Build history of the part. All positions in model axes, mm. A direction names the side the tool comes from. Give positions to 0.01 mm unless a question says otherwise; leave off trailing zeros. Write each loop counter-clockwise with the first axis right and the second up, starting at its lowest first coordinate (ties: lowest second). Pieces come first, ordered by that corner, then holes.
from build123d import *

# Parameters (mm, degrees)
SKETCH1_R               = 9.55
TUBEINTERFACE1_DEPTH    = 5
SKETCH3_R               = 10.922
BODY_DEPTH              = 20.3
BODYCHAMFER_SIZE        = 0.2
SKETCH4_W               = 10
SKETCH4_H               = 75
FLATS_DEPTH             = 12.7
SKETCH5_R               = 7.9375
MOUNTTHREAD1_DEPTH      = 12.7
MOUNTTHREADCHAMFER_SIZE = 1.2
SKETCH17_W              = 2.8
SKETCH17_H              = 5
SKETCH8_R               = 3.5
THRUBORE_DEPTH          = 42.019265815
THRUBORE2_DEPTH         = 38
SKETCH16_R              = 4.639
PORT2_DEPTH             = 10.922
PORT2_DRAFT             = -2
SKETCH26_W              = 2.2
SKETCH26_H              = 0.0127


with BuildPart() as part:
    # Sketch1 → TubeInterface1 (new body)
    with BuildSketch(Plane.XY):
        Circle(SKETCH1_R)
    extrude(amount=TUBEINTERFACE1_DEPTH)

    # Sketch3 → Body (add)
    with BuildSketch(Plane.XY.offset(5)):
        Circle(SKETCH3_R)
    extrude(amount=BODY_DEPTH)

    # BodyChamfer
    bodychamfer_edges = [part.edges().sort_by_distance(p)[0] for p in [
        (-10.922, 0, 25.3),
    ]]
    chamfer(bodychamfer_edges, length=BODYCHAMFER_SIZE)

    # Sketch4 → Flats (cut)
    with BuildSketch(Plane.XY.offset(25.3)):
        with Locations((-14.5, 0)):
            Rectangle(SKETCH4_W, SKETCH4_H)
        with Locations((14.5, 0)):
            Rectangle(SKETCH4_W, SKETCH4_H)
    extrude(amount=-FLATS_DEPTH, mode=Mode.SUBTRACT)

    # Sketch5 → MountThread1 (add)
    with BuildSketch(Plane.XY.offset(25.3)):
        Circle(SKETCH5_R)
    extrude(amount=MOUNTTHREAD1_DEPTH)

    # MountThreadChamfer
    mountthreadchamfer_edges = [part.edges().sort_by_distance(p)[0] for p in [
        (-7.9375, 0, 38),
    ]]
    chamfer(mountthreadchamfer_edges, length=MOUNTTHREADCHAMFER_SIZE)

    # Sketch17 → Cut-Revolve1 (revolve, cut)
    with BuildSketch(Plane(origin=(0, 0, 0), x_dir=(0, 0, -1), z_dir=(1, 0, 0)), mode=Mode.PRIVATE) as cut_revolve1_sk:
        with Locations((-28.9, 9.5)):
            Rectangle(SKETCH17_W, SKETCH17_H)
    revolve(cut_revolve1_sk.sketch.rotate(Axis((0, 0, 0), (0, 0, 1)), 119.564121408), axis=Axis((0, 0, 0), (0, 0, 1)), mode=Mode.SUBTRACT)

    # Sketch8 → ThruBore (cut, through all)
    with BuildSketch(Plane.XY):
        Circle(SKETCH8_R)
    extrude(amount=THRUBORE_DEPTH, mode=Mode.SUBTRACT)

    # Sketch21 → ThruBore2 (cut)
    with BuildSketch(Plane.XY.offset(38)):
        Polygon((3.2, -1.847520861), (3.2, 1.847520861), (0, 3.695041723), (-3.2, 1.847520861), (-3.2, -1.847520861), (0, -3.695041723), align=None)
    extrude(amount=-THRUBORE2_DEPTH, mode=Mode.SUBTRACT)

    # Sketch25 → Chamfer1 (revolve, cut)
    with BuildSketch(Plane(origin=(0, 0, 0), x_dir=(0, 0, -1), z_dir=(1, 0, 0)), mode=Mode.PRIVATE) as chamfer1_sk:
        Polygon((-38, 3.7), (-36, 1.7), (-38, 1.7), align=None)
        Polygon((-38, -3.7), (-36, -1.7), (-38, -1.7), align=None)
    revolve(chamfer1_sk.sketch.rotate(Axis((0, 0, 23.920180356), (0, 0, -1)), 240.435878592), axis=Axis((0, 0, 23.920180356), (0, 0, -1)), mode=Mode.SUBTRACT)


with BuildPart() as port2_tool:
    # Sketch16 → Port2 (with draft: the straight prism first)
    with BuildSketch(Plane(origin=(0, 10.922, 15.05), x_dir=(1, 0, 0), z_dir=(0, 1, 0))):
        with Locations((0, 1.25)):
            Circle(SKETCH16_R)
    extrude(amount=-PORT2_DEPTH)
    # Port2: the draft: its side faces are tilted about the plane it starts from
    port2_sides = [port2_tool.faces().sort_by_distance(p)[0] for p in [
        (-4.639, 5.461, 13.8),
    ]]
    draft(port2_sides, Plane(origin=(0, 10.922, 15.05), x_dir=(1, 0, 0), z_dir=(0, 1, 0)), PORT2_DRAFT)


with BuildPart() as part_1:
    add(part.part)

    # Port2: cut by port2_tool
    add(port2_tool.part, mode=Mode.SUBTRACT)

    # Sketch22 → PortChamfer (revolve, cut)
    with BuildSketch(Plane(origin=(0, 0, 0), x_dir=(0, 0, -1), z_dir=(1, 0, 0)), mode=Mode.PRIVATE) as portchamfer_sk:
        Polygon((-15.8, 10.922), (-19.5, 10.922), (-15.8, 7.222), align=None)
    revolve(portchamfer_sk.sketch.rotate(Axis((0, 0, 13.8), (0, -1, 0)), 90), axis=Axis((0, 0, 13.8), (0, -1, 0)), mode=Mode.SUBTRACT)

    # Sketch23 → RodCoverCrimp (revolve, cut)
    with BuildSketch(Plane(origin=(0, 0, 0), x_dir=(0, 0, -1), z_dir=(1, 0, 0)), mode=Mode.PRIVATE) as rodcovercrimp_sk:
        Polygon((-7.5, 13.6), (-5, 13.6), (-5, 10.2), (-5.5, 10.2), (-7.1, 8.6), (-7.5, 8.6), align=None)
    revolve(rodcovercrimp_sk.sketch.rotate(Axis((0, 0, 0), (0, 0, -1)), 90), axis=Axis((0, 0, 0), (0, 0, -1)), mode=Mode.SUBTRACT)

    # Sketch24 → TubeInterfaceCrimp (revolve, cut)
    with BuildSketch(Plane(origin=(0, 0, 0), x_dir=(0, 0, -1), z_dir=(1, 0, 0)), mode=Mode.PRIVATE) as tubeinterfacecrimp_sk:
        with BuildLine():
            Line((-5, 14.7), (-5, 8.9))
            ThreePointArc((-5, 8.9), (-4.912132034, 8.687867966), (-4.7, 8.6))
            Line((-4.7, 8.6), (-4.1, 8.6))
            Line((-4.1, 8.6), (-3.15, 9.55))
            Line((-3.15, 9.55), (-1, 9.55))
            Line((-1, 9.55), (0, 8.972649731))
            Line((0, 8.972649731), (0, 14.7))
            Line((0, 14.7), (-5, 14.7))
        make_face()
    revolve(tubeinterfacecrimp_sk.sketch.rotate(Axis((0, 0, 0), (0, 0, -1)), 90), axis=Axis((0, 0, 0), (0, 0, -1)), mode=Mode.SUBTRACT)

    # Sketch26 → Cut-Revolve2 (revolve, cut)
    with BuildSketch(Plane(origin=(0, 0, 0), x_dir=(0, 0, -1), z_dir=(1, 0, 0)), mode=Mode.PRIVATE) as cut_revolve2_sk:
        with Locations((-26.4, 7.93115)):
            Rectangle(SKETCH26_W, SKETCH26_H)
    revolve(cut_revolve2_sk.sketch.rotate(Axis((0, 0, 38), (0, 0, 1)), 90), axis=Axis((0, 0, 38), (0, 0, 1)), mode=Mode.SUBTRACT)


solid = part_1.part
(1) 3-axis set-ups, long thin cutter, end or side, ignore diameter. For faces 1 (the face through (-10, 0, 12.6)), 2 (the face through (0, -4, 0)), 3 (the face through (3.5, 0, 18.6)), 4 (the face through (-8.59, -0.38, 4.4)): which of +Z, -Z, +X, -X, +Y, -Y reach the whole face in a straight line?
(2) Saw through at B-B, the plane z = 32.5. List the corners of the cut face in (x, y) (1 decimal).
(3) Saw through at A-A, the plane z = 24.5. List the corners of the cut face in (x, y).
(4) Probe line 1 (Z direction, x = -8.75, y = 2.75); line 2 (X direction, y = 1.5, z = 18); line 3 (Z direction, x = -0.25, y = -9.25). List the from-to ranges inside material, lowest first.
(5) Drop flat-ended pins along their axis: pin 1 (8.5 mm diameter, centred on y = 0, z = 18, fed in from -X); pin 2 (2 mm diameter, centred on x = -3, z = 26, fed in from -Y); pin 3 (0.7 mm diameter, centred on x = -10, y = -0.5, fed in from +Z). Give the stop position or say it passes through.
(6) Mould opens along Y. For faces 5 (the face through (5.8, -5.4, 26.4)), 6 (the face through (1.8, 3, 27.3)), 7 (the face through (-6.5, 4.9, 25.3)) say: +Y half, -Y half, draft (parallel to the pull), parting line (faces both ways), or undercut.
(7) Saw through at C-C, the plane z = 13.8. List the corners of the cut face in (x, y), plus the area to 3 significant figures.
Computed values:
1. face 1: +Z, -X, +Y, -Y
1. face 2: -Z, +X, -X, +Y, -Y
1. face 3: +Z, -Z
1. face 4: none
2. outline: circle Ø15.9 at (0, 0); hole (-3.2, -1.8) - (-2.8, -2.1) arc R3.5 ccw to (-0.4, -3.5) - (0, -3.7) - (0.4, -3.5) arc R3.5 ccw to (2.8, -2.1) - (3.2, -1.8) - (3.2, -1.4) arc R3.5 ccw to (3.2, 1.4) - (3.2, 1.8) - (2.8, 2.1) arc R3.5 ccw to (0.4, 3.5) - (0, 3.7) - (-0.4, 3.5) arc R3.5 ccw to (-2.8, 2.1) - (-3.2, 1.8) - (-3.2, 1.4) arc R3.5 ccw to (-3.2, -1.4) - close
3. outline: (-9.5, -5.39) arc R10.92 ccw to (9.5, -5.39) - (9.5, 5.39) arc R10.92 ccw to (-9.5, 5.39) - close; hole (-3.2, -1.85) - (-2.83, -2.06) arc R3.5 ccw to (-0.37, -3.48) - (0, -3.7) - (0.37, -3.48) arc R3.5 ccw to (2.83, -2.06) - (3.2, -1.85) - (3.2, -1.42) arc R3.5 ccw to (3.2, 1.42) - (3.2, 1.85) - (2.83, 2.06) arc R3.5 ccw to (0.37, 3.48) - (0, 3.7) - (-0.37, 3.48) arc R3.5 ccw to (-2.83, 2.06) - (-3.2, 1.85) - (-3.2, 1.42) arc R3.5 ccw to (-3.2, -1.42) - close
4. line 1: z = 0.35 to 3.53, 5 to 6.53, 7.5 to 25.3
4. line 2: x = -9.5 to -3.2, 3.2 to 9.5
4. line 3: z = 0.49 to 3.45, 5 to 6.45, 7.5 to 25.3
5. pin 1: stops at x = -9.5
5. pin 2: stops at y = -10.62
5. pin 3: stops at z = 12.6
6. face 5: parting line
6. face 6: undercut
6. face 7: draft
7. outline: (-9.5, -5.39) arc R10.92 ccw to (9.5, -5.39) - (9.5, 5.39) arc R10.92 ccw to (4.66, 9.88) - (4.6, 9.82) - (4.26, 0) - (3.5, 0) arc R3.5 cw to (3.2, -1.42) - (3.2, -1.85) - (2.83, -2.06) arc R3.5 cw to (0.37, -3.48) - (0, -3.7) - (-0.37, -3.48) arc R3.5 cw to (-2.83, -2.06) - (-3.2, -1.85) - (-3.2, -1.42) arc R3.5 cw to (-3.5, 0) - (-4.26, 0) - (-4.6, 9.82) - (-4.66, 9.88) arc R10.92 ccw to (-9.5, 5.39) - close
7. area: 241 mm2
